from build123d import *

# Parameters (mm, degrees)
SKETCH1_W           = 240
SKETCH1_H           = 240
SKETCH1_R           = 2.55
BOSS_EXTRUDE1_DEPTH = 10
SKETCH2_W           = 200
SKETCH2_H           = 200
CUT_EXTRUDE1_DEPTH  = 5
FILLET1_R           = 10
SKETCH3_W           = 50
SKETCH3_H           = 20
CUT_EXTRUDE2_DEPTH  = 150


with BuildPart() as part:
    # Sketch1 → Boss-Extrude1 (new body)
    with BuildSketch(Plane.XY):
        Rectangle(SKETCH1_W, SKETCH1_H)
        with Locations((-110, 110)):
            Circle(SKETCH1_R, mode=Mode.SUBTRACT)
        with Locations(Location((110, 110, 0), (0, 0, 180))):
            Circle(SKETCH1_R, mode=Mode.SUBTRACT)
        with Locations((110, -110)):
            Circle(SKETCH1_R, mode=Mode.SUBTRACT)
        with Locations(Location((-110, -110, 0), (0, 0, 180))):
            Circle(SKETCH1_R, mode=Mode.SUBTRACT)
        with Locations((-70, 110)):
            Circle(SKETCH1_R, mode=Mode.SUBTRACT)
        with Locations(Location((-70, -110, 0), (0, 0, 180))):
            Circle(SKETCH1_R, mode=Mode.SUBTRACT)
        with Locations((-50, 110)):
            Circle(SKETCH1_R, mode=Mode.SUBTRACT)
        with Locations(Location((-50, -110, 0), (0, 0, 180))):
            Circle(SKETCH1_R, mode=Mode.SUBTRACT)
    extrude(amount=BOSS_EXTRUDE1_DEPTH)

    # Sketch2 → Cut-Extrude1 (cut)
    with BuildSketch(Plane.XY.offset(10)):
        Rectangle(SKETCH2_W, SKETCH2_H)
    extrude(amount=-CUT_EXTRUDE1_DEPTH, mode=Mode.SUBTRACT)

    # Fillet1
    # the kernel refuses this fillet: 10 mm, written as the material it adds along each edge
    with BuildSketch(Plane(origin=(100, -100, 5), x_dir=(0, 0, 1), z_dir=(0, 1, 0)), Plane(origin=(-100, -100, 5), x_dir=(0, 0, 1), z_dir=(1, 0, 0)), Plane(origin=(-100, 100, 5), x_dir=(0, 0, 1), z_dir=(0, -1, 0)), Plane(origin=(100, 100, 5), x_dir=(0, 0, 1), z_dir=(-1, 0, 0))) as fillet1_piece_1:
        with BuildLine():
            CenterArc((10, -8.660254038), FILLET1_R, 120, 60)
            Line((0, -8.660254038), (0, 0))
            Line((0, 0), (5, 0))
        make_face()
    extrude(amount=200)

    # Sketch3 → Cut-Extrude2 (cut)
    with BuildSketch(Plane.XY.offset(10)):
        with Locations((75, -110)):
            Rectangle(SKETCH3_W, SKETCH3_H)
    extrude(amount=-CUT_EXTRUDE2_DEPTH, mode=Mode.SUBTRACT)


solid = part.part
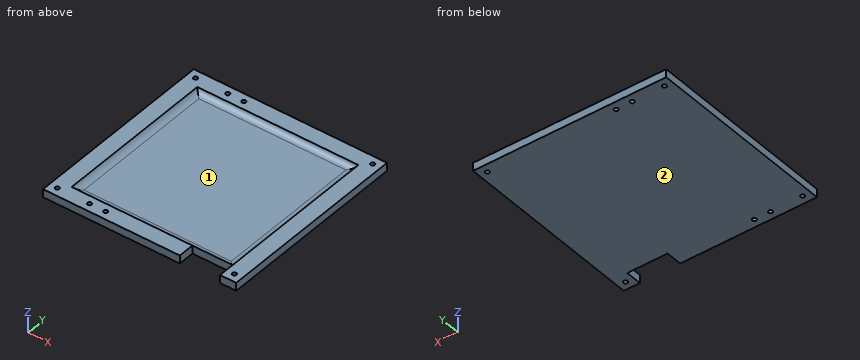
Design review of the part built by this model. Coordinates are the model's own, in mm. Face numbers are marked on the shaded views. Give positions to 0.01 mm unless a question says otherwise; leave off trailing zeros. Order: outer loops, then holes, each group sorted by start corner. A loop starts at its lowest first (then second) coordinate and runs counter-clockwise, first axis right, second up.
1. Add section B-B, the plane z = 2. State how many separate pieces and enclosed holes the cut face has, then the cut area to 3 significant figures.
Solution:
separate pieces: 1
enclosed holes: 8
area: 56,400 mm2
2. To check wall thickness, follow L1, parallel to Y at x = -110, z = 8.25; L2, parallel to Z at x = -34.5, y = -67; L3, parallel to Y at x = 78.5, z = 6.5. State the ranges of each line that lie inside material, in increasing order.
Solution:
L1: y = -120 to -112.55, -107.45 to 107.45, 112.55 to 120
L2: z = 0 to 5
L3: y = -100 to -96.61, 96.61 to 120
3. Mouldability with a two-part tool opening along Y and no side actions: class the marked faces 1 and 2 as +Y half, -Y half, draft (parallel to the pull), parting line (faces both ways), or undercut.
Solution:
face 1: undercut
face 2: draft
4. Add section A-A, the plane y = -86. State the section outline as (x, z) points, then the cut area to 3 significant figures.
Solution:
outline: (-120, 0) - (120, 0) - (120, 10) - (100, 10) arc R10 cw to (91.34, 5) - (-91.34, 5) arc R10 cw to (-100, 10) - (-120, 10) - close
area: 1,430 mm2
5. Add section D-D, the plane x = 95.5. State the section outline as (y, z) points, then the cut area to 3 significant figures.
Solution:
outline: (-100, 0) - (120, 0) - (120, 10) - (100, 10) arc R10 cw to (95.5, 5.91) - (-95.5, 5.91) arc R10 cw to (-100, 10) - close
area: 1,400 mm2
